Autodesk Inventor part; units mm, degrees
ref_plane "YZ Plane" through (0, 0, 0) normal (1, 0, 0) x (0, 1, 0)
ref_plane "XZ Plane" through (0, 0, 0) normal (0, 1, 0) x (-1, 0, 0)
ref_plane "XY Plane" through (0, 0, 0) normal (0, 0, 1) x (1, 0, 0)
sketch "Base Profile" plane through (0, 0, 0) normal (0, 1, 0) x (-1, 0, 0)
  line L0 (0, 0) -> (15, 0)
  line L1 (15, 0) -> (15, -15)
  line L2 (15, -15) -> (0, -15)
  line L3 (0, -15) -> (0, 0)
  line L4 (15, 0) -> (31.5, 0)
  line L5 (31.5, 0) -> (31.5, -15)
  line L6 (31.5, -15) -> (15, -15)
  line L7 (15, -15) -> (15, 0)
  dimension "d164" = 15
  dimension "d165" = 15
  dimension "d166" = 16.5
  dimension "d167" = 15
extrude "Stock" add sketch "Base Profile" against normal blind 33
extrude "Top Extrusion Post" add sketch "Base Profile" along normal blind 15 contours L0 L1 L2 L3
extrude "Lower Extrusion Post" add sketch "Base Profile" against normal blind 22.5 from surface at -33 contours L0 L1 L2 L3
sketch "Sketch27" plane through (0, -33, -15) normal (0, 0, -1) x (-1, 0, 0)
  line L0 (0, -22.5) -> (0, 48)
  line L1 (31.5, 0) -> (15, 0)
  line L2 (31.5, 33) -> (31.5, 0)
  line L3 (15, 33) -> (31.5, 33)
  line L4 (15, 33) -> (15, 48)
  line L5 (0, 48) -> (15, 48)
  line L6 (0, 16.5) -> (31.5, 16.5)
  line L7 (0, 7.5) -> (31.5, 7.5)
  line L8 (15, 33) -> (15, 0)
  line L9 (0, -22.5) -> (15, -22.5)
  line L10 (15, 0) -> (15, -22.5)
  point P0 (15, 16.5)
  point P1 (15, 7.5)
  dimension "d247" = 16.5
  dimension "d290" = 7.5
extrude "Lower Half Cut" cut sketch "Sketch27" against normal through all contours L8 L6 L2 L7
sketch "Bottom Profile" plane through (-35, -33, -15) normal (0, -1, 0) x (1, 0, 0)
  line L0 (13.5, 7.5) -> (10, 7.5) construction
  line L1 (13.5, 10.675) -> (10, 10.675)
  line L2 (10, 4.325) -> (13.5, 4.325)
  arc A0 (13.5, 4.325) -> (13.5, 10.675) centre (13.5, 7.5) ccw
  arc A1 (10, 10.675) -> (10, 4.325) centre (10, 7.5) ccw
  line L3 (3.5, 15) -> (3.5, 0)
  line L4 (35, 15) -> (3.5, 15)
  point P0 (11.75, 7.5)
  dimension "d291" = 3.5
  dimension "d292" = 6.35
  dimension "d293" = 6.5
  dimension "d294" = 7.5
extrude "Slot Cut" cut sketch "Bottom Profile" against normal blind 24
sketch "Front Hole Pattern" plane through (0, -33, 0) normal (1, 0, 0) x (0, 0, -1)
  line L0 (0, 0) -> (0, 48)
  circle A0 centre (7.5, 40.5) radius 3.175
  line L1 (0, 48) -> (15, 48)
  circle A1 centre (7.5, 21.25) radius 3.175
  line L2 (15, 0) -> (0, 0)
  circle A2 centre (7.5, -7.5) radius 3.175
  circle A3 centre (7.5, 2.75) radius 3.175
  dimension "d317" = 6.35
  dimension "d318" = 7.5
  dimension "d319" = 7.5
  dimension "d354" = 6.35
  dimension "d356" = 21.25
  dimension "d369" = 6.35
  dimension "d370" = 7.5
  dimension "d371" = 6.35
  dimension "d372" = 2.75
hole "Front Adjustment Hole" at (0, -11.75, -7.5) at (0, -30.25, -7.5) direction (-1, 0, 0) diameter 3.2004 end through all counterbore diameter 6.35 counterbore depth 10.675
hole "Front Mounting Hole" at (0, 7.5, -7.5) at (0, -40.5, -7.5) direction (-1, 0, 0) diameter 3.2004 end through all counterbore diameter 6.35 counterbore depth 10.675
sketch "Sketch33" plane through (0, 15, 0) normal (0, 1, 0) x (1, 0, 0)
  line L0 (-15, 15) -> (-15, 0)
  line L1 (-15, 0) -> (0, 0)
  line L2 (0, 0) -> (0, 15)
  line L3 (0, 15) -> (-15, 15)
  circle A0 centre (-7.5, 7.5) radius 3.175
  dimension "d340" = 6.35
  dimension "d341" = 7.5
  dimension "d342" = 7.5
hole "Top Mounting Hole" at (-7.5, 15, -7.5) direction (0, -1, 0) diameter 3.2004 end through all counterbore diameter 6.35 counterbore depth 61.674
fillet "Fillet2" radius 6.35 2 edges at (-31.5, -29.25, 0) (-31.5, -8.25, 0)
equation "\"d164\" = extrusionWidth"
equation "\"d165\" = extrusionWidth"
equation "\"d166\" = idlerLength"
equation "\"d167\" = d165"
equation "\"d168\" = extrusionOffset"
equation "\"extrusionWidth\" = 15"
equation "\"idlerLength\" = 16.5"
equation "\"bearingOffsetFromBottom\" = 7.5"
equation "\"extrusionOffset\" = 33"
equation "\"bearingStackHeight\" = 9"
equation "\"bearingSlotLength\" = 3.5"
equation "\"bearingClearance\" = 13"
equation "\"pinSupportLength\" = 2"
properties part number "A Idler" material "Aluminum 6061"
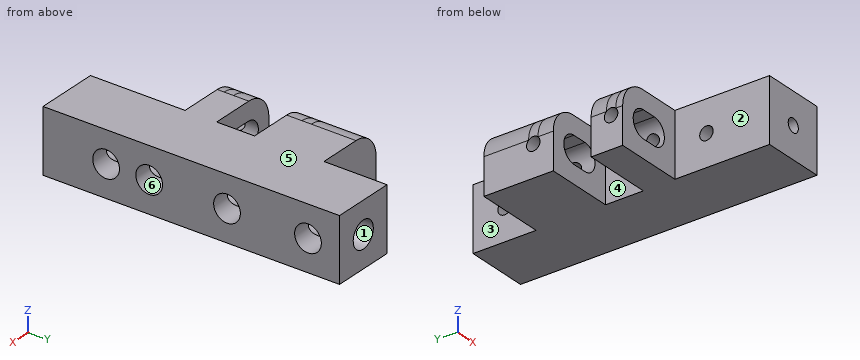
Here's how the part is built. I have some questions about the finished solid (model axes, mm). Face numbers are marked on the shaded views. A direction names the side the tool comes from. Coordinates: 2 decimals unless noted, no trailing zeros. Order: outer loops, then holes, each group sorted by start corner. A loop starts at its lowest first (then second) coordinate and runs counter-clockwise, first axis right, second up. Notation, with made-up numbers: M -16.75,-8 L -0.75,-8 A19 cw -0.75,26 Z; hole C -28.75,54 d3. An arc over 180 degrees is marked long. Answer as CSV lines item,"result".
Item 1: For pin 1 (3 mm diameter, centred on x = -23.5, z = -8, fed in from -Y); pin 2 (5 mm diameter, centred on y = -40.5, z = -7.5, fed in from -X); pin 3 (4 mm diameter, centred on y = -11.75, z = -7.5, fed in from +X) (3 decimals), each with a flat end and sliding along its axis, tell me the tip position at first contact or that it passes through.
Results found:
pin 1,"y = -9"
pin 2,"x = -15"
pin 3,"x = -10.675"
Item 2: On a 3-axis mill with a long thin cutter (end or side, diameter ignored), from which of +Z, -Z, +X, -X, +Y, -Y can I reach the whole of each face in a straight line? I mean the marked faces 1, 2 and 3. Say none if no direction works.
Results found:
face 1,"+Y"
face 2,"+Z, -Z, -X, -Y"
face 3,"+Z, -Z, -X, +Y"
Item 3: If I drill on line 1 (Y direction, x = -17, z = -7.5); line 2 (Y direction, x = -2, z = -7.5) (3 decimals); line 3 (X direction, y = -2.25, z = -7.5) (3 decimals), over which ranges is the centre line in solid material (lowest first)?
Results found:
line 1,"-33 to -31.85, -28.65 to -25.5, -16.5 to -13.35, -10.15 to 0"
line 2,"-55.5 to -43.675, -37.325 to -33.425, -27.075 to -14.925, -8.575 to 4.325, 10.675 to 15"
line 3,"-31.5 to -10.675, -4.325 to 0"
Item 4: Imagine slicing it at C-C on z = -10. Give the number of separate pieces and of enclosed holes in the cut face, plus the area to 3 significant figures.
Results found:
separate pieces,"6"
enclosed holes,"0"
area,"995 mm2"
Item 5: Imagine slicing it at B-B on y = -51. Write out the boundary of the cut face in (x, z).
Results found:
outline,"M -15,-15 L 0,-15 L 0,0 L -15,0 Z; hole C -7.5,-7.5 d3.2"
Item 6: Imagine slicing it at A-A on x = -3. Write out the boundary of the cut face in (y, z) (3 decimals), plus the area to 3 significant figures.
Results found:
outline,"M -55.5,-15 L 15,-15 L 15,0 L -55.5,0 Z; hole C -40.5,-7.5 d6.35; hole C -30.25,-7.5 d6.35; hole C -11.75,-7.5 d6.35; hole C 7.5,-7.5 d6.35"
area,"931 mm2"
Item 7: We'd pull the mould along Z, two halves only. Please class the marked faces 4, 5 and 6: +Z half, -Z half, draft (parallel to the pull), parting line (faces both ways), or undercut.
Results found:
face 4,"draft"
face 5,"+Z half"
face 6,"undercut"
Item 8: Imagine slicing it at D-D on y = -22. Write out the boundary of the cut face in (x, z) (3 decimals), plus the area to 3 significant figures.
Results found:
outline,"M -15,-15 L 0,-15 L 0,0 L -15,0 Z; hole C -7.5,-7.5 d6.35"
area,"193 mm2"
